Answer from the drawing. Dimensions are ordinates in mm from the lowest x, y and z of the part. Coordinates: 2 decimals unless noted, no trailing zeros. Order: outer loops, then holes, each group sorted by start corner. A loop starts at its lowest first (then second) coordinate and runs counter-clockwise, first axis right, second up. Notation, with made-up numbers: M -23.75,41 L 25.25,41 A18 ccw 25.25,53 Z; hole C 74,-18 d1. An arc over 180 degrees is marked long. Use a Markdown table: item, result.
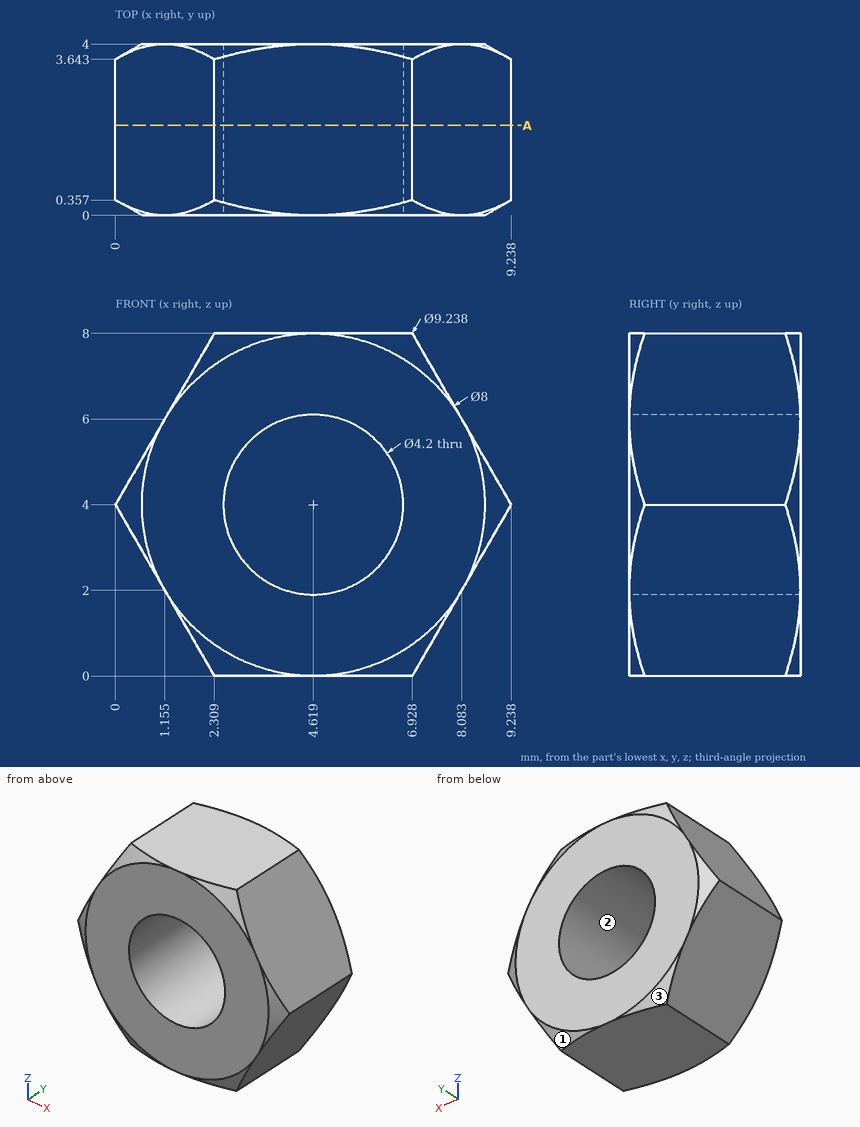
(1) A cutting plane is placed at A-A (y = 2.1). Determine the outline of the cut face in (x, z).
Conclusion:
| item | result |
|---|---|
| outline | M 0,4 L 2.31,0 L 6.93,0 L 9.24,4 L 6.93,8 L 2.31,8 Z; hole C 4.62,4 d4.2 |
(2) Determine the mould class of the marked faces 1, 2 and 3 for opening direction X: pulls with the +X half, pulls with the -X half, needs draft (parallel to the pull), parting line crosses it, or undercut.
Conclusion:
| item | result |
|---|---|
| face 1 | pulls with the +X half |
| face 2 | undercut |
| face 3 | pulls with the -X half |
(3) Straight lines are drawn through the part: L1, parallel to Z at x = 5.25, y = 0.35; L2, parallel to X at y = 3.45, z = 2.25 (1 decimal); L3, parallel to Z at x = 6.25, y = 1.8 (1 decimal). For each, find the intervals that lie inside material, in ascending order.
Conclusion:
| item | result |
|---|---|
| L1 | 0 to 2, 6 to 8 |
| L2 | 1 to 3.5, 5.8 to 8.2 |
| L3 | 0 to 2.7, 5.3 to 8 |
(4) Given P1, Ø1.5, axis at x = 8, y = 0.5, coming from the +Z side (1 decimal), flat-ended and moving along its own axis, determine where the tip first touches the part or whether it passes through.
Conclusion:
| item | result |
|---|---|
| P1 | z = 7.4 |
